For this review, take the finished solid that the model builds, in its own axes (mm). Face numbers are marked on the shaded views. A direction names the side the tool comes from. Coordinates: 2 decimals unless noted, no trailing zeros. Loops run counter-clockwise (first coordinate to the right, second up) from the corner with the lowest first, then second, coordinate; pieces in that order, holes last.
1. Take a section at A-A, the plane y = 28. State the section outline as (x, z) points.
2. Machinability: for the marked faces 5 and 6, which of the approach directions +Z, -Z, +X, -X, +Y, -Y give a long, thin tool a straight path to every point of the face, cutting with its end or side? Answer none if there is none.
3. Mouldability with a two-part tool opening along Z and no side actions: class the marked faces 1, 2, 3 and 4 as pulls with the +Z half, pulls with the -Z half, needs draft (parallel to the pull), parting line crosses it, or undercut.
4. Clearance check with a flat-ended pin moving along its axis: P1, Ø5, axis at x = 46.5, z = -103.5, coming from the +Y side. State where the tip first meets the part, or that it passes through.
5. To check wall thickness, follow probe 1 along Z at (x, y) = (42.5, 16); probe 2 along X at (y, z) = (12.5, -82); probe 3 along Y at (x, z) = (18.5, -208.5). State the ranges of each line that lie inside material, in increasing order.
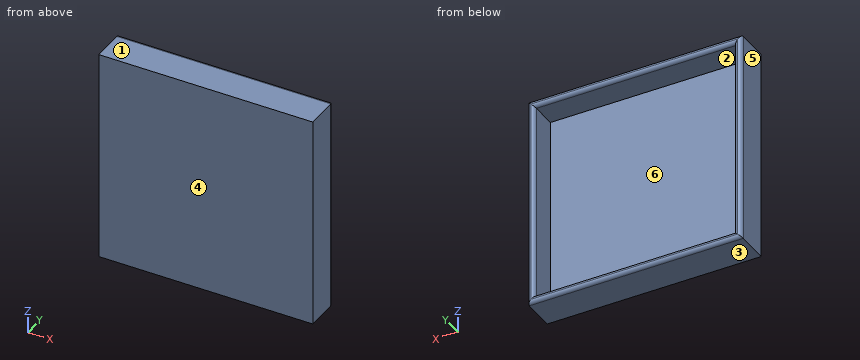
```python
from build123d import *

# Parameters (mm, degrees)
SKETCH1_W           = 300
SKETCH1_H           = 300
BOSS_EXTRUDE1_DEPTH = 50
SKETCH2_W           = 280
SKETCH2_H           = 280
CUT_EXTRUDE1_DEPTH  = 40
FILLET1_R           = 5


with BuildPart() as part:
    # Sketch1 → Boss-Extrude1 (new body)
    with BuildSketch(Plane(origin=(0, 0, 0), x_dir=(1, 0, 0), z_dir=(0, 1, 0))):
        with Locations((150, 150)):
            Rectangle(SKETCH1_W, SKETCH1_H)
    extrude(amount=BOSS_EXTRUDE1_DEPTH)

    # Sketch2 → Cut-Extrude1 (cut)
    with BuildSketch(Plane(origin=(0, 50, 0), x_dir=(1, 0, 0), z_dir=(0, 1, 0))):
        with Locations((150, 150)):
            Rectangle(SKETCH2_W, SKETCH2_H)
    extrude(amount=-CUT_EXTRUDE1_DEPTH, mode=Mode.SUBTRACT)

    # Fillet1
    fillet1_edges = [part.edges().sort_by_distance(p)[0] for p in [
        (300, 50, -150),
        (150, 50, 0),
        (290, 50, -150),
        (150, 50, -290),
        (10, 50, -150),
        (150, 50, -10),
        (0, 50, -150),
        (150, 50, -300),
    ]]
    fillet(fillet1_edges, radius=FILLET1_R - 0.0001)  # a hair under: the kernel refuses the full size


solid = part.part
```
Results list:
1. outline: (0, -300) - (300, -300) - (300, 0) - (0, 0) - close; hole (10, -290) - (290, -290) - (290, -10) - (10, -10) - close
2. face 5: +Z, -Z, -X, +Y, -Y
2. face 6: +Y
3. face 1: pulls with the +Z half
3. face 2: undercut
3. face 3: pulls with the -Z half
3. face 4: needs draft
4. P1: stops at y = 10
5. probe 1: z = -300 to -290, -10 to 0
5. probe 2: x = 0 to 10, 290 to 300
5. probe 3: y = 0 to 10
